The drawing under review shows one solid part. Ordinate dimensions are in mm from its lowest x, y, z. Round coordinates to 2 decimals unless told otherwise and drop trailing zeros. Write each loop counter-clockwise with the first axis right and the second up, starting at its lowest first coordinate (ties: lowest second). Pieces come first, ordered by that corner, then holes. Notation, with made-up numbers: (47.25, 80.5) -> (60.25, 80.5) arc R14 ccw to (60.25, 94.5) -> close; hole circle Ø6 at (-21, 9). An arc over 180 degrees is marked (long way). Answer in a Markdown table with one row per item. Add a question column.
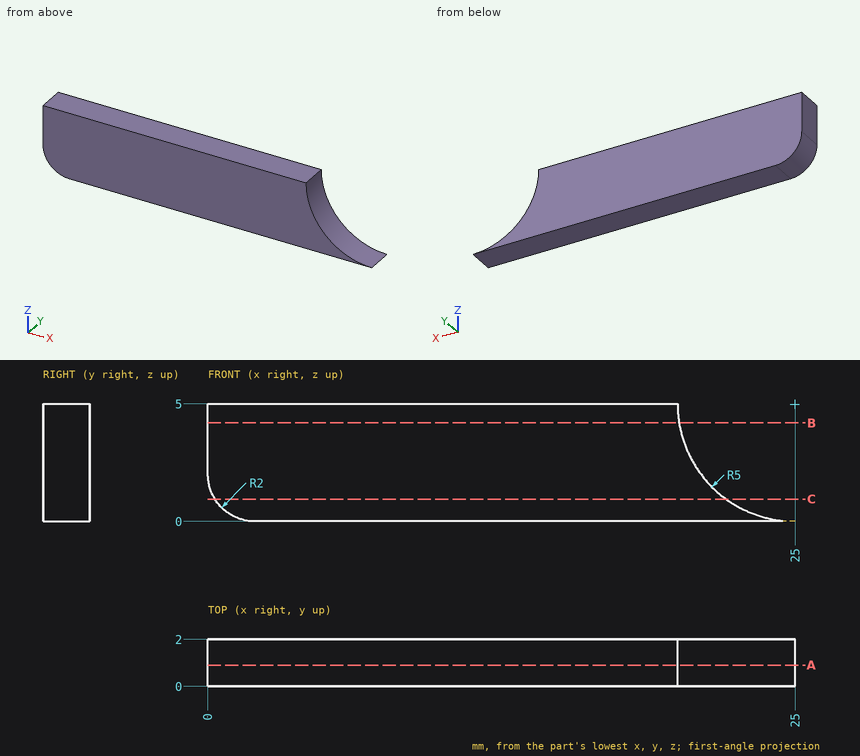
1. Add section B-B on z = 4.2. Write out the cut boundary in (x, y).
2. Add section A-A on y = 0.9. Write out the cut boundary in (x, z), plus the area to 3 significant figures.
3. Add section C-C on z = 0.95. Write out the cut boundary in (x, y).
4. For L1, parallel to X at y = 0.6, z = 0.5; L2, parallel to X at y = 0.7, z = 1.5; L3, parallel to Z at x = 21.25, y = 1.25, list the stretches that pass through material, from the lowest coordinate up.
Filled in:
| question | item | result |
|---|---|---|
| 1 | outline | (0, 0) -> (20.06, 0) -> (20.06, 2) -> (0, 2) -> close |
| 2 | outline | (0, 2) arc R2 ccw to (2, 0) -> (25, 0) arc R5 cw to (20, 5) -> (0, 5) -> close |
| 2 | area | 105 mm² |
| 3 | outline | (0.3, 0) -> (22.07, 0) -> (22.07, 2) -> (0.3, 2) -> close |
| 4 | L1 | 0.68 to 22.82 |
| 4 | L2 | 0.06 to 21.43 |
| 4 | L3 | 0 to 1.69 |
